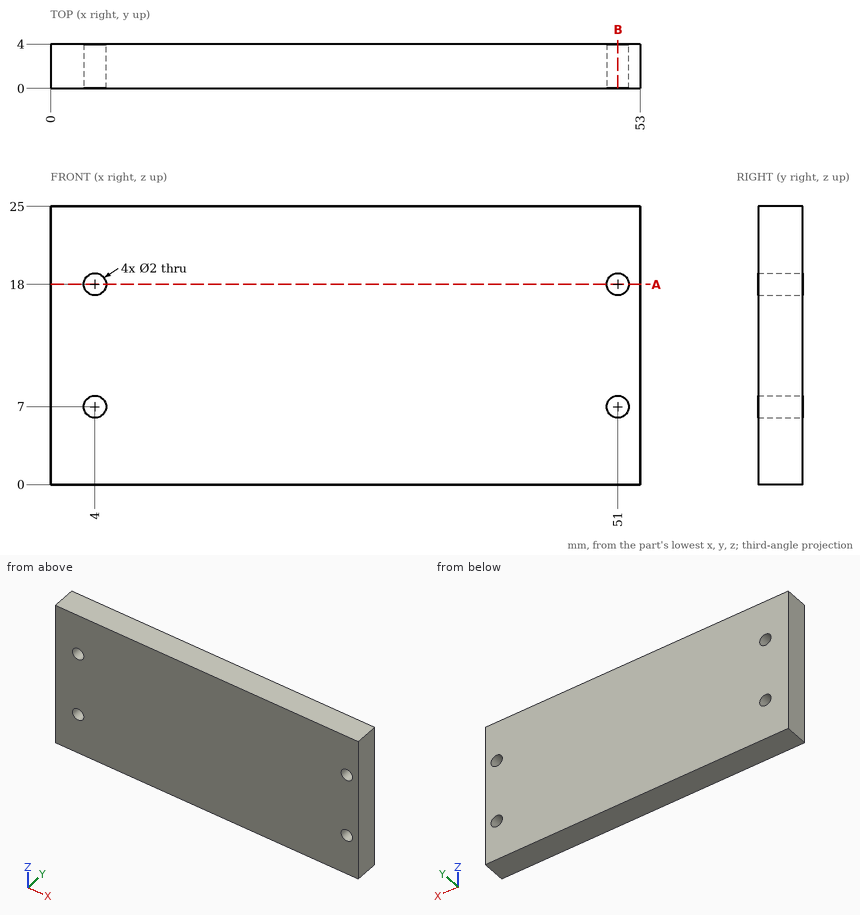
Check sheet for the drawn part. Datum: minimum x, y, z corner. Units: mm. Round coordinates to 2 decimals unless told otherwise and drop trailing zeros. Order: outer loops, then holes, each group sorted by start corner. A loop starts at its lowest first (then second) coordinate and runs counter-clockwise, first axis right, second up.
(1) Cross-section at B-B, the plane x = 51. Enter the section's corners in (y, z), and give its area (3 significant figures).
(2) Go/stop test with a flat-tipped pin: P1, Ø1.8, axis at x = 4, z = 18, coming from the -Y side. Record where the tip stops, or that it passes through.
(3) Scan lines: probe 1 along Z at (x, y) = (4, 1.6); probe 2 along X at (y, z) = (1, 18.75). Record each from-to range of solid material in increasing order.
(4) Cross-section at A-A, the plane z = 18. Enter the section's corners in (x, y), and give its area (3 significant figures).
Check sheet entries:
1. outline: (0, 0) - (4, 0) - (4, 6) - (0, 6) - close; (0, 8) - (4, 8) - (4, 17) - (0, 17) - close; (0, 19) - (4, 19) - (4, 25) - (0, 25) - close
1. area: 84.0 mm2
2. P1: passes through
3. probe 1: z = 0 to 6, 8 to 17, 19 to 25
3. probe 2: x = 0 to 3.34, 4.66 to 50.34, 51.66 to 53
4. outline: (0, 0) - (3, 0) - (3, 4) - (0, 4) - close; (5, 0) - (50, 0) - (50, 4) - (5, 4) - close; (52, 0) - (53, 0) - (53, 4) - (52, 4) - close
4. area: 196 mm2
